```python
from build123d import *

# Parameters (mm, degrees)
F1_DEPTH = 20
F2_W     = 20.4075463116
F2_H     = 3.4
F3_DEPTH = 25
F4_R     = 1.69999


# Not quite as in the source:
# - a fillet or chamfer is up to 0.001 mm smaller than in the source, because OpenCascade refuses the exact size


with BuildPart() as f1:
    # F0 (on Top) → F1 (new body)
    with BuildSketch(Plane.XY):
        Polygon((-2.8867513459, 0), (0, 0), (30, 0), (30, 5), (0, 5), (-15, 30.9807621135), (-19.3301270189, 28.4807621135), align=None)
    extrude(amount=F1_DEPTH)

    # F2 (on face) → F3 (cut)
    with BuildSketch(Plane.XZ):
        with Locations((13.9012318105, 10)):
            Rectangle(F2_W, F2_H)
    extrude(amount=-F3_DEPTH, mode=Mode.SUBTRACT)

    # F4 (radius 1.7 in the source; OpenCascade refuses exactly that, so slightly less here)
    f4_edges = [f1.edges().sort_by_distance(p)[0] for p in [
        (3.697459, 2.5, 8.3),
        (3.697459, 2.5, 11.7),
        (24.105005, 2.5, 11.7),
        (24.105005, 2.5, 8.3),
        (30, 2.5, 20),
        (30, 2.5, 0),
        (-17.165064, 29.730762, 20),
        (-17.165064, 29.730762, 0),
    ]]
    fillet(f4_edges, radius=F4_R)


solid = f1.part
```
Geometry check sheet. Reference: the model listing, model coordinates, mm. A direction names the side the tool comes from. Round coordinates to 2 decimals unless told otherwise and drop trailing zeros. Loops run counter-clockwise (first coordinate to the right, second up) from the corner with the lowest first, then second, coordinate; pieces in that order, holes last. Notation, with made-up numbers: M 71.5,48.25 L 120.5,48.25 A26 cw 120.5,65.25 Z; hole C 19.5,-21.5 d1. An arc over 180 degrees is marked long. Return JSON: item names as keys, results as strings. Group by question number.
(1) Section check C-C, the plane x = 2. Enter the section's corners in (y, z), and give its area (3 significant figures).
(2) Section check A-A, the plane x = 8. Enter the section's corners in (y, z), and give its area (3 significant figures).
(3) Section check D-D, the plane y = 24. Enter the section's corners in (x, z), and give its area (3 significant figures).
(4) Section check B-B, the plane z = 3. Enter the section's corners in (x, y).
(5) Mould release check, pull along X, two halves, no side actions. Record for faces 1 (the face through (29.489, 2.535, 19.515)), 2 (the face through (14, 2, 8.3)), 3 (the face through (15, 5, 8)): pulls with the +X half, pulls with the -X half, needs draft (parallel to the pull), parting line crosses it, or undercut.
(6) Scan lines: line 1 along Y through (x, z) = (3, 8.75); line 2 along X through (y, z) = (27, 10.25); line 3 along X through (y, z) = (24.5, 11). Record each from-to range of solid material in increasing order. Write a range as [from, to].
(7) Set-up check for faces 4 (the face through (29.489, 2.535, 0.485)), 5 (the face through (4.182, 2.535, 8.811)): record each of +Z, -Z, +X, -X, +Y, -Y from which the full face is reachable in a straight line by a thin tool's end or side.
(8) Go/stop test with flat-tipped pins: pin 1 (8 mm diameter, centred on y = 10, z = 3, fed in from -X); pin 2 (6 mm diameter, centred on x = 14.5, z = 12, fed in from +Y); pin 3 (8 mm diameter, centred on y = 5, z = 13, fed in from -X). Record where each tip stops, or that it passes through.
Data:
{
 "1": {"outline": "M 0,0 L 5,0 L 5,20 L 0,20 Z", "area": "100 mm²"},
 "2": {"outline": "M 0,0 L 5,0 L 5,8.3 L 0,8.3 Z; M 0,11.7 L 5,11.7 L 5,20 L 0,20 Z", "area": "83.0 mm²"},
 "3": {"outline": "M -16.74,0 L -10.97,0 L -10.97,20 L -16.74,20 Z", "area": "115 mm²"},
 "4": {"outline": "M -19.33,28.48 L -2.89,0 L 30,0 L 30,5 L 0,5 L -15,30.98 Z"},
 "5": {"face 1": "pulls with the +X half", "face 2": "undercut", "face 3": "needs draft"},
 "6": {"line 1": "[0, 5]", "line 2": "[-18.48, -12.7]", "line 3": "[-17.03, -11.26]"},
 "7": {"face 4": "-Z, +X, +Y, -Y", "face 5": "+Y, -Y"},
 "8": {"pin 1": "x = -10.97", "pin 2": "y = 5", "pin 3": "x = -8.08"}
}
